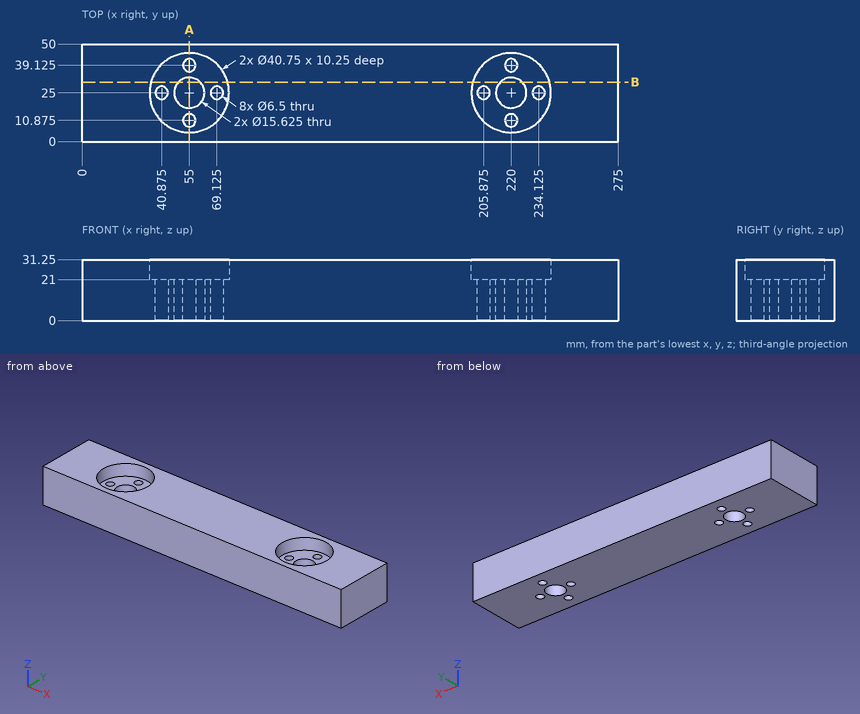
Verification items for this drawing (mm, ordinates from the low corner). Coordinates: 2 decimals unless noted, no trailing zeros. Loops run counter-clockwise (first coordinate to the right, second up) from the corner with the lowest first, then second, coordinate; pieces in that order, holes last.
Item 1: Thickness scan on line 1 (X direction, y = 25, z = 25.25) (3 decimals); line 2 (Y direction, x = 55, z = 12.5) (1 decimal); line 3 (X direction, y = 36, z = 28). Record the ranges inside material, lowest first.
Item 2: Go/stop test with flat-tipped pins: pin 1 Ø7.5 at (x, y) = (55, 39.125) entering from -Z; pin 2 Ø6 at (x, y) = (60.5, 22) entering from +Z; pin 3 Ø5 at (x, y) = (205.875, 25) entering from -Z. Record where each tip stops, or that it passes through.
Item 3: Sectioned sample at B-B, the plane y = 30.5. Record the boundary of the cut face in (x, z), then the cut area to 3 significant figures.
Item 4: Sectioned sample at A-A, the plane x = 55. Count the separate pieces of the cut face and the enclosed holes in it, then the cut area to 3 significant figures.
Check result:
1. line 1: x = 0 to 34.625, 75.375 to 199.625, 240.375 to 275
1. line 2: y = 0 to 7.6, 14.1 to 17.2, 32.8 to 35.9, 42.4 to 50
1. line 3: x = 0 to 37.85, 72.15 to 202.85, 237.15 to 275
2. pin 1: stops at z = 0
2. pin 2: stops at z = 21
2. pin 3: passes through
3. outline: (0, 0) - (49.45, 0) - (49.45, 21) - (35.38, 21) - (35.38, 31.25) - (0, 31.25) - close; (60.55, 0) - (214.45, 0) - (214.45, 21) - (200.38, 21) - (200.38, 31.25) - (74.62, 31.25) - (74.62, 21) - (60.55, 21) - close; (225.55, 0) - (275, 0) - (275, 31.25) - (239.62, 31.25) - (239.62, 21) - (225.55, 21) - close
3. area: 7,320 mm2
4. separate pieces: 4
4. enclosed holes: 0
4. area: 544 mm2
